Source: CAD feature listing. Evaluate the final solid. Frame: model axes, mm. A direction names the side the tool comes from. Round coordinates to 2 decimals unless told otherwise and drop trailing zeros. Loops run counter-clockwise (first coordinate to the right, second up) from the corner with the lowest first, then second, coordinate; pieces in that order, holes last. Notation, with made-up numbers: (51, 79) - (92, 79) arc R21 cw to (92, 98) - close; hole circle Ø5 at (20, 7). An arc over 180 degrees is marked (long way). One line per question, with ' | ' between items. Start each with the question number.
1. Cut plane A-A (x = 6.25). Return loops of the section in (y, z), then the cut area to 3 significant figures.
2. Pin query (flat end, axial travel): pin 1 (5 mm diameter, centred on y = -1, z = 4.5, fed in from -X); pin 2 (0.6 mm diameter, centred on x = 13.5, z = 5, fed in from -Y); pin 3 (0.6 mm diameter, centred on x = 12, y = -5, fed in from +Z); pin 4 (3.5 mm diameter, centred on y = -1.5, z = -2, fed in from -X). Return the tip coordinate at first contact, or that it passes through.
3. Access query for faces 1 (the flat face through (0, 0, 0)), 2 (the cylindrical face through (5, 1, 0)). Directions: +Z, -Z, +X, -X, +Y, -Y. A direction counts if a zero-diameter tool reaches every point of the face in a straight line with its end or side. Return the directions, or none.
4. Ray query, line 1 (X direction, y = -3.5, z = 4.25); line 2 (X direction, y = -1.5, z = 5.5); line 3 (Y direction, x = 12.75, z = -3). Return the intervals inside material, ascending.
```python
from build123d import *

# Parameters (mm, degrees)
CUT_EXTRUDE1_DEPTH = 22.725560982
CIRPATTERN1_START  = 10
CIRPATTERN1_DEPTH  = 6.163521733


# Read off the part's stored shape, not the designer's step: CirPattern1
with BuildPart() as part:
    # Sketch2 → Revolve1 (revolve)
    with BuildSketch(Plane.XY, mode=Mode.PRIVATE) as revolve1_sk:
        with BuildLine():
            Line((0, 0), (0, 1))
            Line((0, 1), (10, 1))
            Line((10, 1), (10, 6))
            Line((10, 6), (16, 6))
            ThreePointArc((16, 6), (16.748287591, 3.041381265), (17, 0))
            Line((17, 0), (0, 0))
        make_face()
    revolve(revolve1_sk.sketch.rotate(Axis((0, 0, 0), (1, 0, 0)), 90), axis=Axis((0, 0, 0), (1, 0, 0)))

    # Sketch3 → Cut-Extrude1 (cut, through all)
    with BuildSketch(Plane(origin=(20, 0, 0), x_dir=(0, 0, -1), z_dir=(1, 0, 0))):
        with BuildLine():
            Line((0, 5.5), (-0.284771266, 5.9932383))
            ThreePointArc((-0.284771266, 5.9932383), (0, 6), (0.284771266, 5.9932383))
            Line((0.284771266, 5.9932383), (0, 5.5))
        make_face()
    extrude(amount=-CUT_EXTRUDE1_DEPTH, mode=Mode.SUBTRACT)

    # CirPattern1 outline → CirPattern1 (cut)
    with BuildSketch(Plane.YZ.offset(CIRPATTERN1_START)):
        with BuildLine():
            ThreePointArc((-2.75, 5.332682252), (-3, 5.196152423), (-3.2432383, 5.047910986))
            Line((-3.2432383, 5.047910986), (-2.75, 4.763139721))
            Line((-2.75, 4.763139721), (-2.75, 5.332682252))
        make_face()
        with BuildLine():
            Line((5.416442642, -0.955064977), (5.852737532, -1.321159859))
            ThreePointArc((5.852737532, -1.321159859), (5.908846518, -1.041889066), (5.951637555, -0.760269959))
            Line((5.951637555, -0.760269959), (5.416442642, -0.955064977))
        make_face()
        with BuildLine():
            Line((5.168309414, -1.881110788), (5.534404296, -2.317405679))
            ThreePointArc((5.534404296, -2.317405679), (5.638155724, -2.05212086), (5.729199314, -1.782210766))
            Line((5.729199314, -1.782210766), (5.168309414, -1.881110788))
        make_face()
        with BuildLine():
            Line((4.763139721, -2.75), (5.047910986, -3.2432383))
            ThreePointArc((5.047910986, -3.2432383), (5.196152422, -3), (5.332682252, -2.75))
            Line((5.332682252, -2.75), (4.763139721, -2.75))
        make_face()
        with BuildLine():
            Line((4.213244437, -3.535331853), (4.408039455, -4.070526767))
            ThreePointArc((4.408039455, -4.070526767), (4.596266658, -3.856725658), (4.774134337, -3.634231876))
            Line((4.774134337, -3.634231876), (4.213244437, -3.535331853))
        make_face()
        with BuildLine():
            Line((3.535331853, -4.213244437), (3.634231876, -4.774134337))
            ThreePointArc((3.634231876, -4.774134337), (3.856725658, -4.596266658), (4.070526767, -4.408039455))
            Line((4.070526767, -4.408039455), (3.535331853, -4.213244437))
        make_face()
        with BuildLine():
            Line((2.75, -4.763139721), (2.75, -5.332682252))
            ThreePointArc((2.75, -5.332682252), (3, -5.196152422), (3.2432383, -5.047910986))
            Line((3.2432383, -5.047910986), (2.75, -4.763139721))
        make_face()
        with BuildLine():
            Line((1.881110788, -5.168309414), (1.782210766, -5.729199314))
            ThreePointArc((1.782210766, -5.729199314), (2.05212086, -5.638155724), (2.317405679, -5.534404296))
            Line((2.317405679, -5.534404296), (1.881110788, -5.168309414))
        make_face()
        with BuildLine():
            Line((0.955064977, -5.416442642), (0.760269959, -5.951637555))
            ThreePointArc((0.760269959, -5.951637555), (1.041889066, -5.908846518), (1.321159859, -5.852737532))
            Line((1.321159859, -5.852737532), (0.955064977, -5.416442642))
        make_face()
        with BuildLine():
            Line((0, -5.5), (-0.284771266, -5.9932383))
            ThreePointArc((-0.284771266, -5.9932383), (0, -6), (0.284771266, -5.9932383))
            Line((0.284771266, -5.9932383), (0, -5.5))
        make_face()
        with BuildLine():
            Line((-0.955064977, -5.416442642), (-1.321159859, -5.852737533))
            ThreePointArc((-1.321159859, -5.852737533), (-1.041889066, -5.908846518), (-0.760269959, -5.951637555))
            Line((-0.760269959, -5.951637555), (-0.955064977, -5.416442642))
        make_face()
        with BuildLine():
            Line((-1.881110788, -5.168309414), (-2.317405679, -5.534404297))
            ThreePointArc((-2.317405679, -5.534404297), (-2.05212086, -5.638155725), (-1.782210766, -5.729199314))
            Line((-1.782210766, -5.729199314), (-1.881110788, -5.168309414))
        make_face()
        with BuildLine():
            Line((-2.75, -4.763139721), (-3.2432383, -5.047910986))
            ThreePointArc((-3.2432383, -5.047910986), (-3, -5.196152423), (-2.75, -5.332682252))
            Line((-2.75, -5.332682252), (-2.75, -4.763139721))
        make_face()
        with BuildLine():
            Line((-3.535331853, -4.213244437), (-4.070526767, -4.408039455))
            ThreePointArc((-4.070526767, -4.408039455), (-3.856725658, -4.596266658), (-3.634231876, -4.774134337))
            Line((-3.634231876, -4.774134337), (-3.535331853, -4.213244437))
        make_face()
        with BuildLine():
            Line((-4.213244437, -3.535331853), (-4.774134337, -3.634231876))
            ThreePointArc((-4.774134337, -3.634231876), (-4.596266658, -3.856725658), (-4.408039455, -4.070526767))
            Line((-4.408039455, -4.070526767), (-4.213244437, -3.535331853))
        make_face()
        with BuildLine():
            Line((-4.763139721, -2.75), (-5.332682252, -2.75))
            ThreePointArc((-5.332682252, -2.75), (-5.196152423, -3), (-5.047910986, -3.2432383))
            Line((-5.047910986, -3.2432383), (-4.763139721, -2.75))
        make_face()
        with BuildLine():
            Line((-5.168309414, -1.881110788), (-5.729199315, -1.782210766))
            ThreePointArc((-5.729199315, -1.782210766), (-5.638155725, -2.05212086), (-5.534404297, -2.317405679))
            Line((-5.534404297, -2.317405679), (-5.168309414, -1.881110788))
        make_face()
        with BuildLine():
            Line((-5.416442642, -0.955064977), (-5.951637555, -0.760269959))
            ThreePointArc((-5.951637555, -0.760269959), (-5.908846518, -1.041889066), (-5.852737533, -1.321159859))
            Line((-5.852737533, -1.321159859), (-5.416442642, -0.955064977))
        make_face()
        with BuildLine():
            Line((-5.5, 0), (-5.9932383, 0.284771266))
            ThreePointArc((-5.9932383, 0.284771266), (-6, 0), (-5.9932383, -0.284771266))
            Line((-5.9932383, -0.284771266), (-5.5, 0))
        make_face()
        with BuildLine():
            Line((-5.416442642, 0.955064977), (-5.852737533, 1.321159859))
            ThreePointArc((-5.852737533, 1.321159859), (-5.908846518, 1.041889066), (-5.951637555, 0.760269959))
            Line((-5.951637555, 0.760269959), (-5.416442642, 0.955064977))
        make_face()
        with BuildLine():
            Line((-5.168309414, 1.881110788), (-5.534404297, 2.317405679))
            ThreePointArc((-5.534404297, 2.317405679), (-5.638155725, 2.05212086), (-5.729199315, 1.782210766))
            Line((-5.729199315, 1.782210766), (-5.168309414, 1.881110788))
        make_face()
        with BuildLine():
            Line((-4.763139721, 2.75), (-5.047910986, 3.2432383))
            ThreePointArc((-5.047910986, 3.2432383), (-5.196152423, 3), (-5.332682252, 2.75))
            Line((-5.332682252, 2.75), (-4.763139721, 2.75))
        make_face()
        with BuildLine():
            Line((-4.213244437, 3.535331853), (-4.408039455, 4.070526767))
            ThreePointArc((-4.408039455, 4.070526767), (-4.596266658, 3.856725658), (-4.774134337, 3.634231876))
            Line((-4.774134337, 3.634231876), (-4.213244437, 3.535331853))
        make_face()
        with BuildLine():
            Line((-3.535331853, 4.213244437), (-3.634231876, 4.774134337))
            ThreePointArc((-3.634231876, 4.774134337), (-3.856725658, 4.596266658), (-4.070526767, 4.408039455))
            Line((-4.070526767, 4.408039455), (-3.535331853, 4.213244437))
        make_face()
        with BuildLine():
            ThreePointArc((5.951637555, 0.760269959), (5.908846518, 1.041889066), (5.852737532, 1.321159859))
            Line((5.852737532, 1.321159859), (5.416442642, 0.955064977))
            Line((5.416442642, 0.955064977), (5.951637555, 0.760269959))
        make_face()
        with BuildLine():
            ThreePointArc((5.729199314, 1.782210766), (5.638155724, 2.05212086), (5.534404296, 2.317405679))
            Line((5.534404296, 2.317405679), (5.168309414, 1.881110788))
            Line((5.168309414, 1.881110788), (5.729199314, 1.782210766))
        make_face()
        with BuildLine():
            ThreePointArc((5.332682252, 2.75), (5.196152422, 3), (5.047910986, 3.2432383))
            Line((5.047910986, 3.2432383), (4.763139721, 2.75))
            Line((4.763139721, 2.75), (5.332682252, 2.75))
        make_face()
        with BuildLine():
            ThreePointArc((4.774134337, 3.634231876), (4.596266658, 3.856725658), (4.408039455, 4.070526767))
            Line((4.408039455, 4.070526767), (4.213244437, 3.535331853))
            Line((4.213244437, 3.535331853), (4.774134337, 3.634231876))
        make_face()
        with BuildLine():
            ThreePointArc((4.070526767, 4.408039455), (3.856725658, 4.596266658), (3.634231876, 4.774134337))
            Line((3.634231876, 4.774134337), (3.535331853, 4.213244437))
            Line((3.535331853, 4.213244437), (4.070526767, 4.408039455))
        make_face()
        with BuildLine():
            ThreePointArc((3.2432383, 5.047910986), (3, 5.196152422), (2.75, 5.332682252))
            Line((2.75, 5.332682252), (2.75, 4.763139721))
            Line((2.75, 4.763139721), (3.2432383, 5.047910986))
        make_face()
        with BuildLine():
            ThreePointArc((2.317405679, 5.534404296), (2.05212086, 5.638155724), (1.782210766, 5.729199314))
            Line((1.782210766, 5.729199314), (1.881110788, 5.168309414))
            Line((1.881110788, 5.168309414), (2.317405679, 5.534404296))
        make_face()
        with BuildLine():
            ThreePointArc((1.321159859, 5.852737532), (1.041889066, 5.908846518), (0.760269959, 5.951637555))
            Line((0.760269959, 5.951637555), (0.955064977, 5.416442642))
            Line((0.955064977, 5.416442642), (1.321159859, 5.852737532))
        make_face()
        with BuildLine():
            ThreePointArc((0.284771266, 5.9932383), (0, 6), (-0.284771266, 5.9932383))
            Line((-0.284771266, 5.9932383), (0, 5.5))
            Line((0, 5.5), (0.284771266, 5.9932383))
        make_face()
        with BuildLine():
            ThreePointArc((-0.760269959, 5.951637555), (-1.041889066, 5.908846518), (-1.321159859, 5.852737533))
            Line((-1.321159859, 5.852737533), (-0.955064977, 5.416442642))
            Line((-0.955064977, 5.416442642), (-0.760269959, 5.951637555))
        make_face()
        with BuildLine():
            ThreePointArc((-1.782210766, 5.729199314), (-2.05212086, 5.638155725), (-2.317405679, 5.534404297))
            Line((-2.317405679, 5.534404297), (-1.881110788, 5.168309414))
            Line((-1.881110788, 5.168309414), (-1.782210766, 5.729199314))
        make_face()
    extrude(amount=CIRPATTERN1_DEPTH, mode=Mode.SUBTRACT)


solid = part.part
```
Answers follow:
1) outline: circle Ø2 at (0, 0) | area: 3.14 mm2
2) pin 1: stops at x = 10 | pin 2: stops at y = -3.63 | pin 3: stops at z = 3.63 | pin 4: stops at x = 0
3) face 1: +Z, -Z, -X, +Y, -Y | face 2: -X
4) line 1: x = 10 to 16.16 | line 2: x = 10 to 16.1 | line 3: y = -4.91 to 4.91
